Geometry check sheet. Reference: the model listing, model coordinates, mm. A direction names the side the tool comes from. Round coordinates to 2 decimals unless told otherwise and drop trailing zeros. Write each loop counter-clockwise with the first axis right and the second up, starting at its lowest first coordinate (ties: lowest second). Pieces come first, ordered by that corner, then holes. Notation, with made-up numbers: (-1, -28) - (25, -28) arc R11 ccw to (25, -18) - close; hole circle Ø4 at (10.25, -23.75). An arc over 180 degrees is marked (long way). Return JSON: item names as keys, results as strings.
```python
from build123d import *

# Parameters (mm, degrees)
BOSS_EXTRU_1_DEPTH              = 5
CONG_1_R                        = 1
DIAM_TRE_DU_PER_AGE_5_5_5_5_1_D = 5.5
D_GAGEMENT_M41_D                = 4.5


with BuildPart() as part:
    # Esquisse1 → Boss.-Extru.1 (new, symmetric)
    with BuildSketch(Plane.XY):
        Polygon((0, 0), (10.5, 0), (10.5, -1.5), (-1.5, -1.5), (-1.5, 17.75), (0, 17.75), align=None)
    extrude(amount=BOSS_EXTRU_1_DEPTH, both=True)

    # Congé1
    cong_1_edges = [part.edges().sort_by_distance(p)[0] for p in [
        (0, 0, 0),
        (-1.5, -1.5, 0),
    ]]
    fillet(cong_1_edges, radius=CONG_1_R)

    # Diamètre du perçage Ø5.5 (5.5)1 (through all)
    with Locations(Plane(origin=(0, 0, 0), x_dir=(0, 0, -1), z_dir=(1, 0, 0))):
        with Locations((0, 12)):
            Hole(DIAM_TRE_DU_PER_AGE_5_5_5_5_1_D / 2)

    # Dégagement M41 (through all)
    with Locations(Plane(origin=(0, 0, 0), x_dir=(1, 0, 0), z_dir=(0, 1, 0))):
        with Locations((5.5, 0)):
            Hole(D_GAGEMENT_M41_D / 2)


solid = part.part
```
(1) Material ranges on line 1 along Z through (x, y) = (5.5, -0.25); line 2 along X through (y, z) = (3.75, 4.25); line 3 along Y through (x, z) = (-0.85, 0), recorded low to high. Write a range as [from, to].
Response values:
{"line 1": "z = [-5, -2.25], [2.25, 5]", "line 2": "x = [-1.5, 0]", "line 3": "y = [-1.44, 9.25], [14.75, 17.75]"}
(2) Section check D-D, the plane z = -3.5. Enter the section's corners in (x, y), plus the area to 3 significant figures.
Response values:
{"outline": "(-1.5, -0.5) arc R1 ccw to (-0.5, -1.5) - (10.5, -1.5) - (10.5, 0) - (1, 0) arc R1 cw to (0, 1) - (0, 17.75) - (-1.5, 17.75) - close", "area": "44.6 mm^2"}
(3) Release check for a two-part mould opening along X. For faces 3 (the face through (3.354, -0.761, -0.676)), 4 (the face through (-0.4, 4.6, -5)), 5 (the face through (0.301, 0.285, 0.07)) record: pulls with the +X half, pulls with the -X half, needs draft (parallel to the pull), parting line crosses it, or undercut.
Response values:
{"face 3": "undercut", "face 4": "needs draft", "face 5": "pulls with the +X half"}
(4) Section check C-C, the plane z = 0. Enter the section's corners in (x, y), plus the area to 3 significant figures.
Response values:
{"outline": "(-1.5, -0.5) arc R1 ccw to (-0.5, -1.5) - (3.25, -1.5) - (3.25, 0) - (1, 0) arc R1 cw to (0, 1) - (0, 9.25) - (-1.5, 9.25) - close; (-1.5, 14.75) - (0, 14.75) - (0, 17.75) - (-1.5, 17.75) - close; (7.75, -1.5) - (10.5, -1.5) - (10.5, 0) - (7.75, 0) - close", "area": "29.6 mm^2"}
(5) Gauge pin test, flat ends, axial feed: pin 1 (5 mm diameter, centred on x = 5, z = -1.5, fed in from +Y); pin 2 (1.5 mm diameter, centred on y = 6, z = 0, fed in from +X). Record the tip position at first contact, or that the pin passes through.
Response values:
{"pin 1": "stops at y = 0", "pin 2": "stops at x = 0"}
(6) Section check A-A, the plane x = 5.5. Enter the section's corners in (y, z), plus the area to 3 significant figures.
Response values:
{"outline": "(-1.5, -5) - (0, -5) - (0, -2.25) - (-1.5, -2.25) - close; (-1.5, 2.25) - (0, 2.25) - (0, 5) - (-1.5, 5) - close", "area": "8.25 mm^2"}
(7) Access from +Z, -Z, +X, -X, +Y, -Y to the whole of each face (thin tool, end or side, straight path). Record for faces 1 (the face through (0, 9, 1)), 2 (the face through (-1.215, -1.199, -0.07)).
Response values:
{"face 1": "+Z, -Z, +X, +Y", "face 2": "+Z, -Z, -X, -Y"}
(8) Section check B-B, the plane y = 12. Enter the section's corners in (x, z).
Response values:
{"outline": "(-1.5, -5) - (0, -5) - (0, -2.75) - (-1.5, -2.75) - close; (-1.5, 2.75) - (0, 2.75) - (0, 5) - (-1.5, 5) - close"}
